Geometry: final body of the model. Coordinates: model frame, mm. A direction names the side the tool comes from. Round coordinates to 2 decimals unless told otherwise and drop trailing zeros. Write each loop counter-clockwise with the first axis right and the second up, starting at its lowest first coordinate (ties: lowest second). Pieces come first, ordered by that corner, then holes. Notation, with made-up numbers: M 32.5,15.5 L 82.5,15.5 A13 cw 82.5,25.5 Z; hole C 10.5,54 d7. An arc over 180 degrees is marked long. Use one line per item in the form item = value. Start each with the question number.
Item 1: Ray query, probe 1 along Y at (x, z) = (-150, 140); probe 2 along X at (y, z) = (-1, 122). Return the intervals inside material, ascending.
Item 2: Section query C-C (z = 128). Return loops of the section in (x, y), and give its area (3 significant figures).
Item 3: Pull-direction query (Y, two-part tool) for faces 4 (the cylindrical face through (-34.51, -4.845, 5.053)), 5 (the cylindrical face through (-34.51, -5.536, 5.775)), 6 (the flat face through (-154, -6, 300)); classes: pulls with the +Y half, pulls with the -Y half, needs draft (parallel to the pull), parting line crosses it, or undercut.
Item 4: Section query B-B (y = 0). Return loops of the section in (x, z), and give its area (3 significant figures).
Item 5: Section query A-A (x = -16.5). Return loops of the section in (y, z).
Item 6: Pin query (flat end, axial travel): pin 1 Ø3 at (x, y) = (-87, 5) entering from -Z; pin 2 Ø1.5 at (y, z) = (-2, 84.5) entering from +X; pin 3 Ø4 at (x, y) = (-110, -0.5) entering from -Z; pin 4 Ø1.6 at (y, z) = (-5, -5.5) entering from +X. Return the tip coordinate at first contact, or that it passes through.
Item 7: Reachability of faces 1 (the cylindrical face through (-34.51, 5.536, -5.775)), 2 (the flat face through (0, 4.8, -5.3)), 3 (the cylindrical face through (-156.466, -2.681, 188.46)) from +Z, -Z, +X, -X, +Y, -Y: full face, straight path, thin tool, end or side. Return the list, or none.
from build123d import *

# Parameters (mm, degrees)
SKETCH_2_R          = 8
SKETCH_2_R_2        = 7
CUT_EXTRUDE_1_DEPTH = 70


with BuildPart() as part:
    # По траектории1: sweep along a path in Эскиз1
    with BuildLine(Plane(origin=(0, 0, 0), x_dir=(1, 0, 0), z_dir=(0, 1, 0))) as sweep_1_path:
        Line((-150, -300), (-150, -80))
        ThreePointArc((-150, -80), (-126.568542495, -23.431457505), (-70, 0))
        Line((-70, 0), (0, 0))
    # Эскиз2 → По траектории1 (sweep)
    with BuildSketch(Plane(origin=(0, 0, 0), x_dir=(0, 0, -1), z_dir=(1, 0, 0))):
        Circle(SKETCH_2_R)
        Circle(SKETCH_2_R_2, mode=Mode.SUBTRACT)
    sweep(path=sweep_1_path.line)

    # Эскиз3 → Вырез-Вытянуть1 (cut)
    with BuildSketch(Plane(origin=(0, 0, 0), x_dir=(0, 0, -1), z_dir=(1, 0, 0))):
        Polygon((5.303300859, -6.01040764), (-6.01040764, 5.303300859), (-5.303300859, 6.01040764), (6.01040764, -5.303300859), align=None)
    extrude(amount=-CUT_EXTRUDE_1_DEPTH, mode=Mode.SUBTRACT)


solid = part.part
Working result:
q1.probe_1 = -8 to -7, 7 to 8
q1.probe_2 = -157.94 to -156.93, -143.07 to -142.06
q2.outline = C -150,0 d16; hole C -150,0 d14
q2.area = 47.1 mm²
q3.face_4 = undercut
q3.face_5 = parting line crosses it
q3.face_6 = needs draft
q4.outline = M -158,80 A88 ccw -70,-8 L 0,-8 L 0,-7 L -70,-7 A87 cw -157,80 L -157,300 L -158,300 Z; M -143,80 A73 ccw -70,7 L 0,7 L 0,8 L -70,8 A72 cw -142,80 L -142,300 L -143,300 Z
q4.area = 831 mm²
q5.outline = M -6,-5.29 L -5.29,-4.58 A7 cw 4.58,5.29 L 5.29,6 A8 ccw Z; M -5.29,-6 A8 ccw 6,5.29 L 5.29,4.58 A7 cw -4.58,-5.29 Z
q6.pin_1 = -5.58
q6.pin_2 = -142.1
q6.pin_3 = 0.64
q6.pin_4 = 0
q7.face_1 = +X
q7.face_2 = +Z, -Z, +X, +Y, -Y
q7.face_3 = +Z
